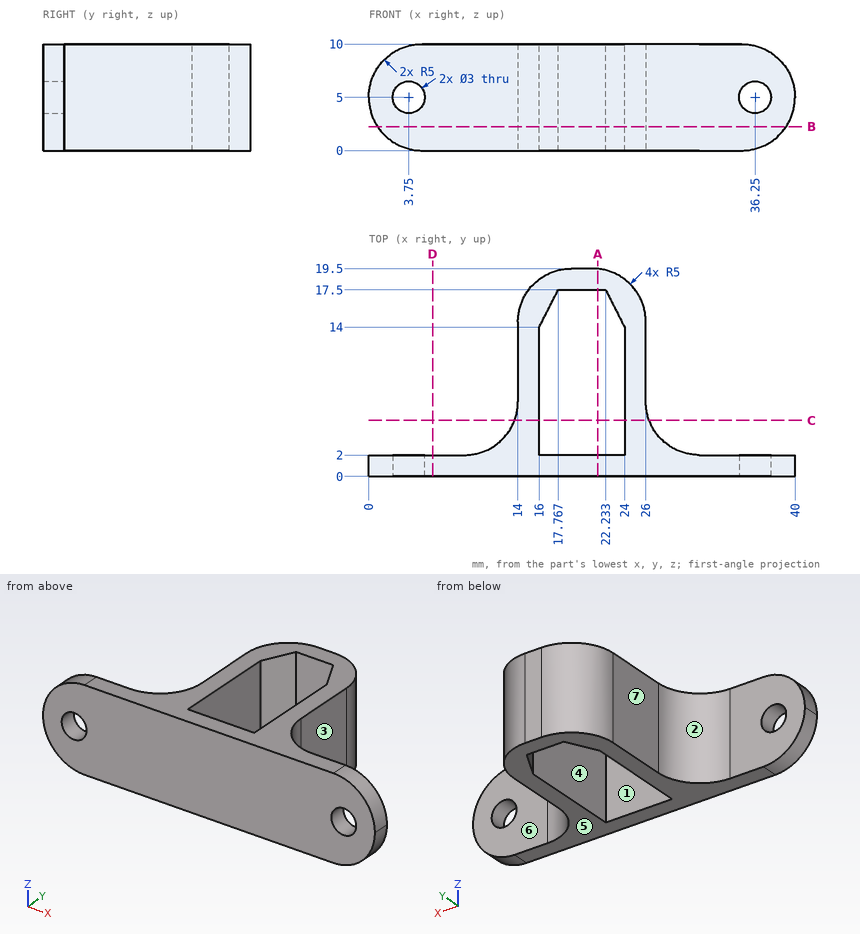
Input: dimensioned drawing with shaded views. Units: mm. Origin: part minimum x, y, z. A direction names the side the tool comes from. Give positions to 0.01 mm unless a question says otherwise; leave off trailing zeros. Write each loop counter-clockwise with the first axis right and the second up, starting at its lowest first coordinate (ties: lowest second). Pieces come first, ordered by that corner, then holes. Notation, with made-up numbers: (68, 53) - (83, 53) arc R27 ccw to (83, 86) - close; hole circle Ø8 at (10.5, 58). An arc over 180 degrees is marked (long way). One line per item, written item: value. Start each with the question number.
Q1. Section query B-B, the plane z = 2.25. Return the cut outline in (x, y) (1 decimal).
Q2. First-contact query: pin 1 Ø2 at (y, z) = (9.5, 1.5) entering from -X; pin 2 Ø3 at (y, z) = (8.5, 7) entering from +X. Flat tips, straight axial feed; report the tip coordinate or a pass-through.
Q3. Draft query along X for the marked faces 1, 2 and 3. Return one class per face: +X half, -X half, draft (parallel to the pull), parting line (faces both ways), or undercut.
Q4. Section query C-C, the plane y = 5.25. Return the cut outline in (x, z).
Q5. Section query A-A, the plane x = 21.5. Return the cut outline in (y, z) (1 decimal).
Q6. Section query D-D, the plane x = 6. Return the cut outline in (y, z).
Q7. Material intervals for probe 1 along X at (y, z) = (8, 5.25); probe 2 along X at (y, z) = (1, 5.25); probe 3 along Y at (x, z) = (7.5, 6.75), sorted ascending. Write a range as from..to.
Q8. Set-up query: the marked faces 4, 5, 6 and 7. Return all of +Z, -Z, +X, -X, +Y, -Y with unobstructed straight access to the full face (end or side cutting, diameter ignored); none if empty.
Answer:
1. outline: (0.8, 0) - (39.2, 0) - (39.2, 2) - (31, 2) arc R5 cw to (26, 7) - (26, 14.5) arc R5 ccw to (21, 19.5) - (19, 19.5) arc R5 ccw to (14, 14.5) - (14, 7) arc R5 cw to (9, 2) - (0.8, 2) - close; hole (16, 2) - (24, 2) - (24, 14) - (22.2, 17.5) - (17.8, 17.5) - (16, 14) - close
2. pin 1: stops at x = 14
2. pin 2: stops at x = 26
3. face 1: undercut
3. face 2: -X half
3. face 3: +X half
4. outline: (13.68, 0) - (16, 0) - (16, 10) - (13.68, 10) - close; (24, 0) - (26.32, 0) - (26.32, 10) - (24, 10) - close
5. outline: (0, 0) - (2, 0) - (2, 10) - (0, 10) - close; (17.5, 0) - (19.5, 0) - (19.5, 10) - (17.5, 10) - close
6. outline: (0, 0) - (2, 0) - (2, 10) - (0, 10) - close
7. probe 1: x = 14..16, 24..26
7. probe 2: x = 0.01..2.27, 5.23..34.77, 37.73..39.99
7. probe 3: y = 0..2
8. face 4: +Z, -Z
8. face 5: -Z, +X, -X, +Y, -Y
8. face 6: +Z, -Z, +X, +Y
8. face 7: +Z, -Z, -X, +Y
